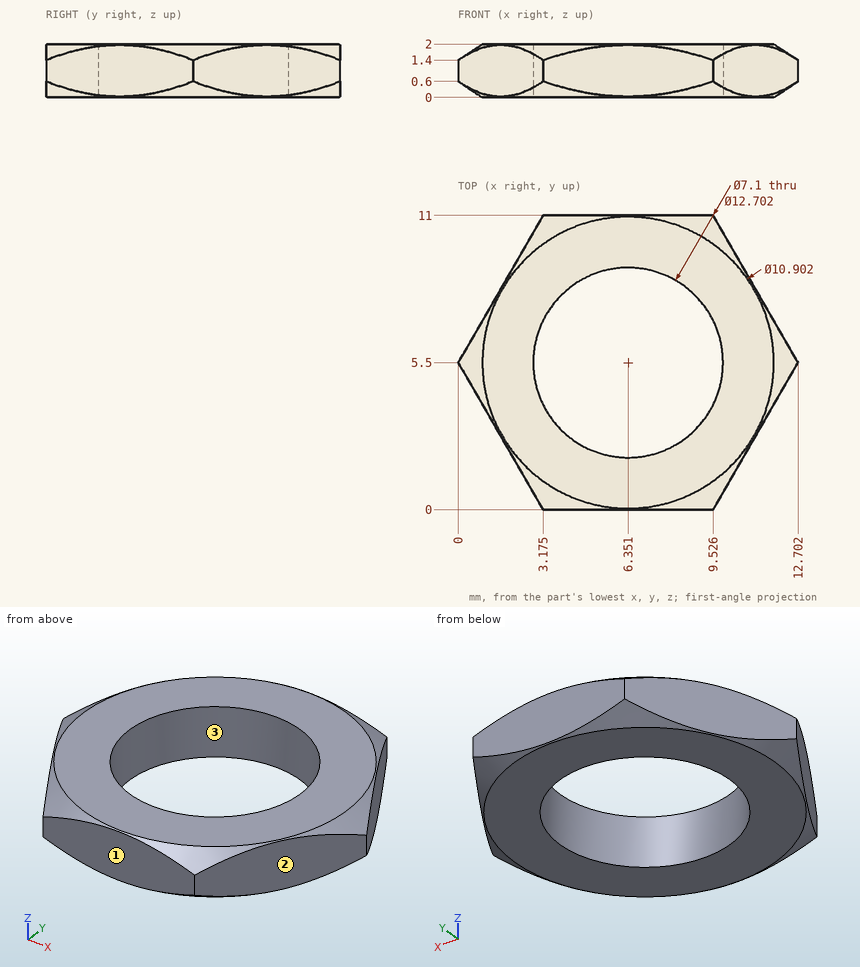
Source: three-view drawing plus pictorial views. Frame: mm from the lowest corner of the part. Coordinates: 2 decimals unless noted, no trailing zeros. One line per item, written item: value. Start each with the question number.
1. Ray query, L1, parallel to Y at x = 8.25, z = 0.8; L2, parallel to Y at x = 3.25, z = 0.1 (1 decimal); L3, parallel to X at y = 8.75, z = 0.45 (1 decimal). Return the intervals inside material, ascending.
2. Mould query, pull axis X, two halves, no side actions, for the marked faces 1, 2 and 3. Classes: pulls with the +X half, pulls with the -X half, needs draft (parallel to the pull), parting line crosses it, or undercut.
3. Contact query for a flat-ended pin moving along its axis: P1, Ø4.5, axis at x = 6.35, y = 5.5, coming from the +Z side. Output: stop coordinate, or through.
Verdict:
1. L1: y = 0 to 2.5, 8.5 to 11
1. L2: y = 0.8 to 3.8, 7.2 to 10.2
1. L3: x = 1.9 to 4.9, 7.8 to 10.8
2. face 1: needs draft
2. face 2: pulls with the +X half
2. face 3: undercut
3. P1: passes through
